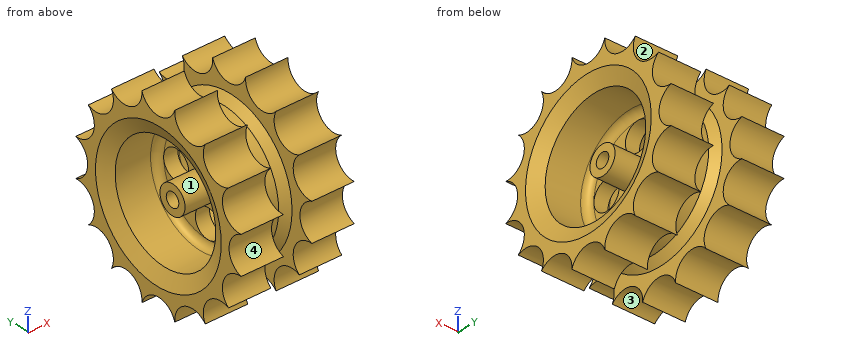
Autodesk Inventor part; units mm, degrees
ref_plane "YZ Plane" through (0, 0, 0) normal (1, 0, 0) x (0, 1, 0)
ref_plane "XZ Plane" through (0, 0, 0) normal (0, 1, 0) x (-1, 0, 0)
ref_plane "XY Plane" through (0, 0, 0) normal (0, 0, 1) x (1, 0, 0)
sketch "Sketch1" plane through (0, 0, 0) normal (0, 0, 1) x (1, 0, 0)
  line L0 (6, 0) -> (6, 2)
  line L1 (6, 0) -> (1, 0)
  line L2 (6, 2) -> (-6, 2)
  line L3 (-6, 2) -> (-6, 0)
  line L4 (-6, 0) -> (-1, 0)
  line L5 (-8, -8) -> (-7, -6)
  line L6 (8, -8) -> (7, -6)
  line L7 (-7, -6) -> (-2, -6)
  line L8 (-1, 0) -> (-1, -5)
  arc A0 (-2, -6) -> (-1, -5) centre (-2, -5) ccw
  line L9 (-2, -8) -> (-1, -7)
  line L10 (-1, -7) -> (1, -7)
  line L11 (1, -7) -> (2, -8)
  line L12 (1, 0) -> (1, -5)
  line L13 (7, -6) -> (2, -6)
  arc A1 (1, -5) -> (2, -6) centre (2, -5) ccw
  line L14 (2, -8) -> (2, -12)
  line L15 (2, -12) -> (8, -12)
  line L16 (8, -12) -> (8, -8)
  line L17 (-8, -8) -> (-8, -12)
  line L18 (-8, -12) -> (-2, -12)
  line L19 (-2, -12) -> (-2, -8)
  point P0 (0, 0)
  dimension "d0" = 6
  dimension "d1" = 2
  dimension "d3" = 5
  dimension "d6" = 12
  dimension "d7" = 2
  dimension "d8" = 5
  dimension "d26" = 5
  dimension "d27" = 5
  dimension "d29" = 5
  dimension "d49" = 2
  dimension "d50" = 1
  dimension "d51" = 4
  dimension "d52" = 4
  dimension "d53" = 6
revolve "Revolution1" add sketch "Sketch1" angle 360 about axis through (6, 2, 0) along (-1, 0, 0)
sketch "Sketch2" plane through (1, 2, 0) normal (1, 0, 0) x (0, 0, -1)
  circle A0 centre (0, 0) radius 8
  line L0 (0, 8) -> (0, 5)
  line L1 (-8, 0) -> (-5, 0)
  line L2 (0, -8) -> (0, -5)
  line L3 (8, 0) -> (5, 0)
  point P0 (0, -2)
  dimension "d15" = 3
  dimension "d16" = 3
  dimension "d17" = 3
  dimension "d18" = 3
hole "Hole1" [suppressed]
sketch "Sketch3" plane through (1, 2, 0) normal (1, 0, 0) x (0, 0, -1)
  line L0 (0, 2.0456) -> (0, 5.0456)
  circle A0 centre (0, 0) radius 2
  line L1 (-2, 0) -> (-5, 0)
  line L2 (0, -2) -> (0, -5)
  line L3 (2, 0) -> (5, 0)
  dimension "d31" = 3
  dimension "d32" = 3
  dimension "d33" = 3
  dimension "d34" = 3
hole "Hole2" at (1, 7.0456, 0) at (1, 2, -5) at (1, -3, 0) at (1, 2, 5) direction (-1, 0, 0) diameter 4 depth 8
sketch "Sketch5" plane through (6, 2, 0) normal (1, 0, 0) x (0, 0, -1)
  point P0 (0, 0)
  point P1 (0, 0)
hole "Hole3" at (6, 2, 0) direction (-1, 0, 0) diameter 2 depth 20
sketch "Sketch7" plane through (8, 2, 0) normal (1, 0, 0) x (0, 0, -1)
  line L0 (0, 0) -> (0, 14)
  line L1 (0, 0) -> (14, 0)
  line L2 (0, 0) -> (0, -14)
  line L3 (0, 0) -> (-14, 0)
  line L4 (0, 0) -> (9.8995, -9.8995)
  line L5 (0, 0) -> (14, 0) construction
  line L6 (0, 0) -> (-9.8995, -9.8995)
  line L7 (0, 0) -> (14, 0) construction
  line L8 (0, 0) -> (-9.8995, 9.8995)
  line L9 (0, 0) -> (14, 0) construction
  line L10 (0, 0) -> (9.8995, 9.8995)
  line L11 (0, 0) -> (12.9343, 5.3576)
  line L12 (0, 0) -> (14, 0) construction
  line L13 (0, 0) -> (12.9343, -5.3576)
  line L14 (0, 0) -> (5.3576, -12.9343)
  line L15 (0, 0) -> (-5.3576, -12.9343)
  line L16 (0, 0) -> (14, 0) construction
  line L17 (0, 0) -> (-12.9343, -5.3576)
  line L18 (0, 0) -> (14, 0) construction
  line L19 (0, 0) -> (-12.9343, 5.3576)
  line L20 (0, 0) -> (14, 0) construction
  line L21 (0, 0) -> (-5.3576, 12.9343)
  line L22 (0, 0) -> (14, 0) construction
  circle A0 centre (0, 0) radius 14
  line L23 (0, 0) -> (5.3576, 12.9343)
  point P0 (0, -2)
  dimension "d54" = 14
  dimension "d55" = 14
  dimension "d56" = 14
  dimension "d57" = 14
  dimension "d58" = 14
  dimension "d59" = 45
  dimension "d60" = 14
  dimension "d61" = 135
  dimension "d62" = 14
  dimension "d63" = 135
  dimension "d64" = 14
  dimension "d65" = 14
  dimension "d66" = 22.5
  dimension "d67" = 14
  dimension "d68" = 14
  dimension "d69" = 14
  dimension "d70" = 112.5
  dimension "d71" = 14
  dimension "d72" = 157.5
  dimension "d73" = 14
  dimension "d74" = 157.5
  dimension "d75" = 14
  dimension "d76" = 112.5
sketch "Sketch8" plane through (8, 2, 0) normal (1, 0, 0) x (0, 0, -1)
  point P0 (0, -2)
hole "Hole4" at (8, 16, 0) at (8, 14.9343, -5.3576) at (8, 11.8995, -9.8995) at (8, 7.3576, -12.9343) at (8, 2, -14) at (8, -3.3576, -12.9343) at (8, -7.8995, -9.8995) at (8, -10.9343, -5.3576) at (8, -12, 0) at (8, -10.9343, 5.3576) at (8, -7.8995, 9.8995) at (8, -3.3576, 12.9343) at (8, 2, 14) at (8, 7.3576, 12.9343) at (8, 11.8995, 9.8995) at (8, 14.9343, 5.3576) direction (-1, 0, 0) diameter 5.5 depth 20
properties part number "Tank drive Wheel"
Can you work these out from the model? Positions are in its coordinate system, mm. Face numbers are marked on the shaded views. A direction names the side the tool comes from. Coordinates: 2 decimals unless noted, no trailing zeros. Loops run counter-clockwise (first coordinate to the right, second up) from the corner with the lowest first, then second, coordinate; pieces in that order, holes last. Notation, with made-up numbers: (54.5, 10.25) - (87.5, 10.25) arc R7 cw to (87.5, 23.25) - close; hole circle Ø5 at (60.25, 51.25). An arc over 180 degrees is marked (long way). Answer as CSV lines item,"result". Start each with the question number.
1) Suppose I cut it at A-A (x = -3.5). Please give me the cut outline in (y, z).
2) Thinking about a two-plate mould opening in Y: for the marked faces 3 and 4, which applies, pulls with the +Y half, pulls with the -Y half, needs draft (parallel to the pull), parting line crosses it, or undercut?
3) For pin 1 (3 mm diameter, centred on y = 2.5, z = -1, fed in from +X); pin 2 (7 mm diameter, centred on y = 3, z = 2.5, fed in from -X); pin 3 (12 mm diameter, centred on y = 5.5, z = 2.5, fed in from -X); pin 4 (3 mm diameter, centred on y = -2, z = 4.5, fed in from +X), each with a flat end and sliding along its axis, tell me the tip position at first contact or that it passes through.
4) Which directions (+Z, -Z, +X, -X, +Y, -Y) give clear straight access to the entire face, cutting with the end or side of a thin tool? Please do the marked faces 1 and 2.
5) I need wall thicknesses on line 1 (Z direction, x = -0.4, y = 2); line 2 (X direction, y = 12, z = 7); line 3 (Y direction, x = 3.75, z = -0.75). Which ranges of each line are inside material? Lowest first, please. Write a range as from..to.
Check result:
1,outline,"(-11.15, -2.62) arc R2.75 cw to (-9.15, -7.45) arc R2.75 cw to (-5.45, -11.15) arc R2.75 cw to (-0.62, -13.15) arc R2.75 cw to (4.62, -13.15) arc R2.75 cw to (9.45, -11.15) arc R2.75 cw to (13.15, -7.45) arc R2.75 cw to (15.15, -2.62) arc R2.75 cw to (15.15, 2.62) arc R2.75 cw to (13.15, 7.45) arc R2.75 cw to (9.45, 11.15) arc R2.75 cw to (4.62, 13.15) arc R2.75 cw to (-0.62, 13.15) arc R2.75 cw to (-5.45, 11.15) arc R2.75 cw to (-9.15, 7.45) arc R2.75 cw to (-11.15, 2.62) arc R2.75 cw to start; circle Ø4 at (2, 0); hole circle Ø16 at (2, 0); hole circle Ø2 at (2, 0)"
2,face 3,"undercut"
2,face 4,"pulls with the -Y half"
3,pin 1,"stops at x = 6"
3,pin 2,"stops at x = -6"
3,pin 3,"stops at x = -8"
3,pin 4,"stops at x = 1.15"
4,face 1,"-X"
4,face 2,"+X, -X"
5,line 1,"z = -9..-7, -3..-1, 1..3, 7..9"
5,line 2,"x = -8..-2, 2..8"
5,line 3,"y = -9.35..-5.96, 0.15..1.34, 2.66..3.85, 9.96..13.35"
